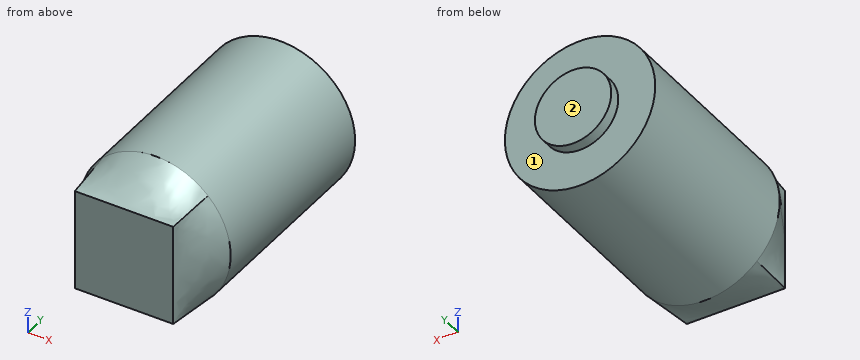
Autodesk Inventor part; units mm, degrees
ref_plane "YZ Plane" through (0, 0, 0) normal (1, 0, 0) x (0, 1, 0)
ref_plane "XZ Plane" through (0, 0, 0) normal (0, 1, 0) x (-1, 0, 0)
ref_plane "XY Plane" through (0, 0, 0) normal (0, 0, 1) x (1, 0, 0)
sketch "Sketch1" plane through (0, 0, 0) normal (0, 1, 0) x (-1, 0, 0)
  circle A0 centre (0, 0) radius 16.3195
  circle A1 centre (0, 0) radius 32.131
  dimension "d0" = 32.639
  dimension "d1" = 64.262
extrude "Extrusion1" add sketch "Sketch1" along normal blind 84.8868 contours A0 | A1
sketch "Sketch2" plane through (0, 84.8868, 0) normal (0, 1, 0) x (1, 0, 0)
  circle A0 centre (0, 0) radius 16.3195
  dimension "d4" = 32.639
extrude "Extrusion2" add sketch "Sketch2" along normal blind 4.7625
sketch "Sketch3" plane through (0, 0, 0) normal (0, -1, 0) x (1, 0, 0)
  circle A0 centre (0, 0) radius 32.131
ref_plane "Work Plane1" through (0, -21.463, 0) normal (0, -1, 0) x (1, 0, 0)
sketch "Sketch4" plane through (0, -21.463, 0) normal (0, -1, 0) x (1, 0, 0)
  line L0 (21.0185, 21.59) -> (-21.0185, 21.59)
  line L1 (-21.0185, 21.59) -> (-21.0185, -21.59)
  line L2 (-21.0185, -21.59) -> (21.0185, -21.59)
  line L3 (21.0185, -21.59) -> (21.0185, 21.59)
  point P0 (0, 0)
  dimension "d8" = 43.18
  dimension "d9" = 42.037
  dimension "d10" = 21.0185
  dimension "d11" = 21.59
loft "Loft1" add profiles "Sketch4" section 1 edges at (32.131, 0, 0)
properties part number "Motor"
Input: part model. Units: mm. Frame: model coordinates. Face numbers are marked on the shaded views. A direction names the side the tool comes from. Coordinates: 2 decimals unless noted, no trailing zeros. Loops run counter-clockwise (first coordinate to the right, second up) from the corner with the lowest first, then second, coordinate; pieces in that order, holes last. Notation, with made-up numbers: (51.25, 31.25) - (77.25, 31.25) arc R18 ccw to (77.25, 56.25) - close; hole circle Ø6 at (74.5, 32). An arc over 180 degrees is marked (long way). Answer in a Markdown table with one row per item. Add a question column.
Item 1: Access query for the marked faces 1 and 2. Directions: +Z, -Z, +X, -X, +Y, -Y. A direction counts if a zero-diameter tool reaches every point of the face in a straight line with its end or side. Return the directions, or none.
Item 2: Line query: line 1 along Y through (x, z) = (-0.5, 21.5); line 2 along Z through (x, y) = (-2.5, 44); line 3 along X through (y, z) = (38, -13). Output: solid intervals per line, ascending. Write a range as [from, to].
Item 3: Contact query for flat-ended pins moving along their axis: P1, Ø1, axis at x = -9, y = 5.5, coming from the -Z side; P2, Ø12, axis at x = 22.5, z = 4.5, coming from the +Y side; P3, Ø3, axis at x = 20.5, y = 22, coming from the -Z side. Output: stop coordinate, or through.
Item 4: Section query A-A on y = 1.5. Return the cut outline in (x, z).
Recorded:
| question | item | result |
|---|---|---|
| 1 | face 1 | +Y |
| 1 | face 2 | +Z, -Z, +X, -X, +Y |
| 2 | line 1 | [-21.46, 84.89] |
| 2 | line 2 | [-32.03, 32.03] |
| 2 | line 3 | [-29.38, 29.38] |
| 3 | P1 | z = -30.99 |
| 3 | P2 | y = 84.89 |
| 3 | P3 | z = -25.91 |
| 4 | outline | circle Ø64.26 at (0, 0) |
